Verification items for the finished model (mm, model axes). Face numbers are marked on the shaded views. A direction names the side the tool comes from. Give positions to 0.01 mm unless a question says otherwise; leave off trailing zeros. Order: outer loops, then holes, each group sorted by start corner. A loop starts at its lowest first (then second) coordinate and runs counter-clockwise, first axis right, second up. Notation, with made-up numbers: (20, 45) -> (78, 45) arc R26 ccw to (78, 73) -> close; hole circle Ø2 at (4, -9). An arc over 180 degrees is marked (long way). One line per question, with ' | ' between items. Start each with the question number.
Q1. Mould release check, pull along Z, two halves, no side actions. Record for the marked faces 3, 4 and 5: released by +Z, released by -Z, zero draft, split by the parting line, or undercut.
Q2. Section check A-A on x = -13.93. Record the cut outline in (y, z).
Q3. Section check C-C on z = 0. Record the cut outline in (x, y).
Q4. Go/stop test with flat-tipped pins: pin 1 (4 mm diameter, centred on y = 16, z = 7, fed in from -X); pin 2 (1.3 mm diameter, centred on y = 2.45, z = -7.525, fed in from -X); pin 3 (1.9 mm diameter, centred on x = -21.455, y = 17.55, fed in from -Z); pin 4 (1.2 mm diameter, centred on x = -21.5, z = -20.5, fed in from -Y). Record where each tip stops, or that it passes through.
Q5. Access from +Z, -Z, +X, -X, +Y, -Y to the whole of each face (thin tool, end or side, straight path). Record for the marked faces 1 and 2.
Q6. Material ranges on probe 1 along Z at (x, y) = (-14.75, 1.5); probe 2 along X at (y, z) = (2, -21); probe 3 along X at (y, z) = (2, -17.5), recorded low to high. Write a range as [from, to].
Q7. Section check B-B on y = 0.5. Record the cut outline in (x, z), plus the area to 3 significant figures.
Q8. Section check D-D on x = -16.5. Record the cut outline in (y, z).
Autodesk Inventor part; units mm, degrees
ref_plane "Work Plane1" through (-24, 20.05, 0) normal (0, 0, 1) x (1, 0, 0)
ref_plane "YZ Plane" through (0, 0, 0) normal (1, 0, 0) x (0, 1, 0)
ref_plane "XZ Plane" through (0, 0, 0) normal (0, 1, 0) x (-1, 0, 0)
sketch "Sketch1" plane through (0, 0, 0) normal (1, 0, 0) x (0, 1, 0)
  line L0 (20.05, 20.25) -> (-20.05, 20.25)
  line L1 (-20.05, 20.25) -> (-20.05, -20.25)
  line L2 (-20.05, -20.25) -> (20.05, -20.25)
  line L3 (20.05, -20.25) -> (20.05, 20.25)
  line L4 (20.05, 20.25) -> (-20.05, -20.25) construction
  line L5 (-20.05, 20.25) -> (20.05, -20.25) construction
  point P0 (0, 0)
  dimension "d0" = 40.1
  dimension "d1" = 40.5
extrude "Plate1" add sketch "Sketch1" along normal blind 1.5
sketch "Sketch2" plane through (0, 20.05, 20.25) normal (0, 0, 1) x (1, 0, 0)
  line L0 (0, -40.1) -> (0, 0)
  line L1 (0, 0) -> (-24, 0)
  line L2 (-24, 0) -> (-24, -40.1)
  line L3 (-24, -40.1) -> (0, -40.1)
edge flange "Flange1" height 25.5 angle 90 thickness 1.5 bend radius 0.31 thickness toward (0, 0, 1) relief tear relief width 1.5 relief depth 0.75 corner gap 0.31 corner form 0 edges at (0, 0, 20.25) (0, 0, -20.25) wall of the first edge with corners at (0, -20.05, 20.25) (0, 20.05, 20.25) (-24, 20.05, 20.25) (-24, -20.05, 20.25)
bend "Bend1"
corner "Corner1"
sketch "Sketch3" plane through (-24, -20.05, 21.75) normal (0, 0, 1) x (1, 0, 0)
  circle A0 centre (10.07, 10) radius 6.4
  line L0 (0, 0) -> (0, 40.1)
  line L1 (23.69, 0) -> (0, 0)
  line L2 (23.69, 0) -> (23.69, 40.1)
  circle A1 centre (10.07, 10) radius 6.9
  line L3 (3.17, 10) -> (0, 10)
  line L4 (16.97, 10) -> (16.97, 0)
  point P0 (24, 20.05)
  point P1 (10.07, 3.1)
  point P2 (10.07, 0)
  dimension "d13" = 0.5
sketch "Sketch4" plane through (-24, -20.05, -21.75) normal (0, 0, -1) x (-1, 0, 0)
  line L0 (-3.17, 10) -> (0, 10)
  line L1 (0, 0) -> (0, 40.1)
  circle A0 centre (-10.07, 10) radius 6.9
  line L2 (-16.97, 10) -> (-16.97, 0)
  line L3 (-23.69, 0) -> (0, 0)
  arc A1 (-17.595, 0) -> (-16.97, 4.9206) centre (-17.595, 2.5) ccw
  point P0 (-24, 20.05)
  dimension "d53" = 5
  dimension "d54" = 2.5
  dimension "d55" = 0.625
extrude "Cut1" cut sketch "Sketch3" against normal blind 1.5 contours A0 | L0 L3 A1 L4 L1 | A1
extrude "Cut2" cut sketch "Sketch4" against normal blind 1.5 contours A0 | L0 L1 L3 L2 A1 A0 | L3 A1 L2
ref_plane "Work Plane1" through (-24, 20.05, 0) normal (0, 0, 1) x (1, 0, 0)
sketch "Sketch5" plane through (-24, 20.05, 21.75) normal (0, 0, 1) x (1, 0, 0)
  circle A0 centre (18.07, -23.2) radius 0.7835
  circle A1 centre (2.07, -23.2) radius 0.7835
  circle A2 centre (3.07, -9.98) radius 0.7835
  circle A3 centre (17.07, -9.98) radius 0.7835
  circle A4 centre (10.07, -2.68) radius 0.7835
  point P0 (24, -20.05)
hole "Hole1" at (-13.93, 17.37, 21.75) at (-20.93, 10.07, 21.75) at (-6.93, 10.07, 21.75) at (-21.93, -3.15, 21.75) at (-5.93, -3.15, 21.75) direction (0, 0, -1) diameter 2.1 depth 1.5
sketch "Sketch6" plane through (-0.31, 20.05, -21.75) normal (0, 0, -1) x (-1, 0, 0)
  circle A0 centre (6.095, -17.6) radius 0.7835
  circle A1 centre (6.095, -2.5) radius 0.7835
  circle A2 centre (21.145, -2.5) radius 0.7835
  circle A3 centre (21.145, -17.6) radius 0.7835
  circle A4 centre (6.095, -37.6) radius 0.7835
  point P0 (-0.31, -20.05)
fillet "Corner Round1" radius 1 4 edges at (-24, 20.05, -21) (-24, -10.05, -21) (-24, 20.05, 21) (-24, -10.05, 21)
hole "Hole3" at (-6.405, 17.55, -21.75) at (-21.455, 17.55, -21.75) at (-6.405, 2.45, -21.75) at (-21.455, 2.45, -21.75) at (-6.405, -17.55, -21.75) direction (0, 0, 1) diameter 2.1 depth 1.5
sketch "Sketch9" plane through (1.5, 0, 0) normal (1, 0, 0) x (0, 0, -1)
  circle A0 centre (7.525, 17.55) radius 0.7835
  circle A1 centre (-7.525, 17.55) radius 0.7835
  circle A2 centre (-7.525, 2.45) radius 0.7835
  circle A3 centre (7.525, 2.45) radius 0.7835
  circle A4 centre (7.525, -17.55) radius 0.7835
  circle A5 centre (-7.525, -17.55) radius 0.7835
  point P0 (0, 0)
hole "Hole4" at (1.5, 17.55, 7.525) at (1.5, 17.55, -7.525) at (1.5, 2.45, 7.525) at (1.5, 2.45, -7.525) at (1.5, -17.55, 7.525) at (1.5, -17.55, -7.525) direction (-1, 0, 0) diameter 2.1 end through all
sketch "Sketch10" plane through (1.5, 0, 0) normal (1, 0, 0) x (0, 0, -1)
  circle A0 centre (0, -10.05) radius 6.4
  circle A1 centre (0, -10.05) radius 6.8
  point P0 (0, 0)
  dimension "d50" = 0.4
extrude "Extrusion1" cut sketch "Sketch10" against normal through all contours A0 | A1
equation "\"d14\" = Thickness"
equation "\"d16\" = Thickness"
equation "\"d23\" = Thickness"
equation "\"d41\" = Thickness"
equation "\"d48\" = Thickness"
equation "\"d2\" = Thickness"
equation "\"d3\" = BendReliefWidth"
equation "\"d4\" = BendReliefDepth"
equation "\"d5\" = MinimumRemnant"
equation "\"d6\" = TransitionRadius"
equation "\"d9\" = BendRadius"
equation "\"d10\" = CornerReliefSize"
equation "\"d11\" = GapSize"
equation "\"d12\" = JacobiRadiusSize"
equation "\"BendReliefWidth\" = Thickness"
equation "\"BendReliefDepth\" = 0.5 * Thickness"
equation "\"CornerReliefSize\" = 4 * Thickness"
equation "\"MinimumRemnant\" = 2 * Thickness"
equation "\"TransitionRadius\" = BendRadius"
equation "\"JacobiRadiusSize\" = BendRadius"
equation "\"GapSize\" = Thickness"
properties part number "axis_3_top_frame" material "Aluminum 6061-AHC"
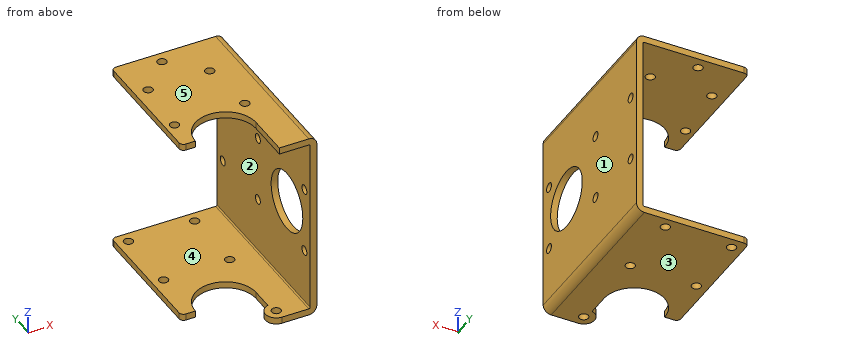
Filled in:
1) face 3: released by -Z | face 4: undercut | face 5: released by +Z
2) outline: (-3.15, -21.75) -> (20.05, -21.75) -> (20.05, -20.25) -> (-3.15, -20.25) -> close; (-3.15, 20.25) -> (16.32, 20.25) -> (16.32, 21.75) -> (-3.15, 21.75) -> close; (18.42, 20.25) -> (20.05, 20.25) -> (20.05, 21.75) -> (18.42, 21.75) -> close
3) outline: (0, -20.05) -> (1.5, -20.05) -> (1.5, -16.85) -> (0, -16.85) -> close; (0, -3.25) -> (1.5, -3.25) -> (1.5, 20.05) -> (0, 20.05) -> close
4) pin 1: x = 0 | pin 2: through | pin 3: z = 20.25 | pin 4: y = -10.05
5) face 1: +Z, -Z, +X, +Y, -Y | face 2: -X, +Y, -Y
6) probe 1: [-21.75, -20.25], [20.25, 21.75] | probe 2: [-24, -22.4], [-20.51, -7.35], [-5.46, 1.16] | probe 3: [0, 1.5]
7) outline: (-24, -21.75) -> (-0.31, -21.75) arc R1.81 ccw to (1.5, -19.94) -> (1.5, 19.94) arc R1.81 ccw to (-0.31, 21.75) -> (-24, 21.75) -> (-24, 20.25) -> (-0.31, 20.25) arc R0.31 cw to (0, 19.94) -> (0, -19.94) arc R0.31 cw to (-0.31, -20.25) -> (-24, -20.25) -> close | area: 136 mm²
8) outline: (-3.65, -21.75) -> (20.05, -21.75) -> (20.05, -20.25) -> (-3.65, -20.25) -> close; (-3.65, 20.25) -> (20.05, 20.25) -> (20.05, 21.75) -> (-3.65, 21.75) -> close
